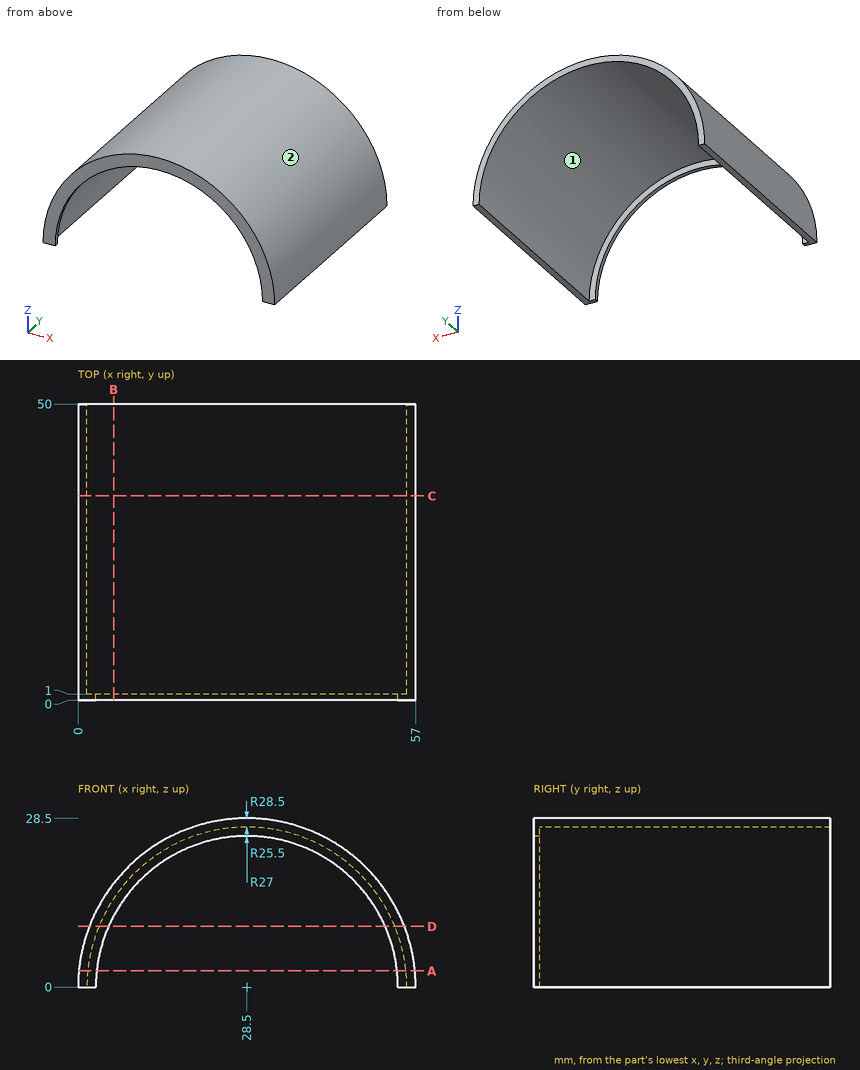
Here's the drawing with two shaded views (mm, measured from the low corner). I have some questions. Coordinates: 2 decimals unless noted, no trailing zeros. Order: outer loops, then holes, each group sorted by start corner. A loop starts at its lowest first (then second) coordinate and runs counter-clockwise, first axis right, second up. Notation, with made-up numbers: M 12.5,-20 L 66.5,-20 A14 cw 66.5,6 Z; hole C 6.25,32.5 d11. An arc over 180 degrees is marked long. Write item = value, one per line.
(1) Suppose I cut it at C-C on y = 34.5. Please give me the cut outline in (x, z).
Results are:
outline = M 0,0 L 1.5,0 A27 cw 55.5,0 L 57,0 A28.5 ccw Z
(2) Suppose I cut it at A-A on z = 2.75. Please give me the cut outline in (x, y).
Results are:
outline = M 0.13,0 L 3.15,0 L 3.15,1 L 1.64,1 L 1.64,50 L 0.13,50 Z; M 53.85,0 L 56.87,0 L 56.87,50 L 55.36,50 L 55.36,1 L 53.85,1 Z
(3) For pin 1 Ø2 at (x, y) = (13.5, 24.5) entering from -Z; pin 2 Ø4 at (x, y) = (47, 31.5) entering from -Z; pin 3 Ø5 at (y, z) = (16.5, 19) entering from -X; pin 4 Ø3 at (x, z) = (50.5, 21) entering from +Y, each with a flat end and sliding along its axis, tell me the tip position at first contact or that it passes through.
Results are:
pin_1 = 21.75
pin_2 = 17.57
pin_3 = 5.26
pin_4 = through
(4) Suppose I cut it at B-B on x = 6. Please give me the cut outline in (y, z).
Results are:
outline = M 0,12 L 1,12 L 1,14.92 L 50,14.92 L 50,17.49 L 0,17.49 Z
(5) I need wall thicknesses on line 1 along X through (y, z) = (23, 10); line 2 along Z through (x, y) = (29, 39); line 3 along X through (y, z) = (35, 12.5). Which ranges of each line are inside material? Lowest first, please. Write a range as [from, to].
Results are:
line_1 = [1.81, 3.42], [53.58, 55.19]
line_2 = [27, 28.5]
line_3 = [2.89, 4.57], [52.43, 54.11]
(6) Suppose I cut it at D-D on z = 10.25. Please give me the cut outline in (x, y).
Results are:
outline = M 1.91,0 L 5.15,0 L 5.15,1 L 3.52,1 L 3.52,50 L 1.91,50 Z; M 51.85,0 L 55.09,0 L 55.09,50 L 53.48,50 L 53.48,1 L 51.85,1 Z
(7) If we mould it in two halves opening along X, with no side actions, what happens to the marked faces 1 and 2? For each: pulls with the +X half, pulls with the -X half, needs draft (parallel to the pull), parting line crosses it, or undercut.
Results are:
face_1 = undercut
face_2 = parting line crosses it
